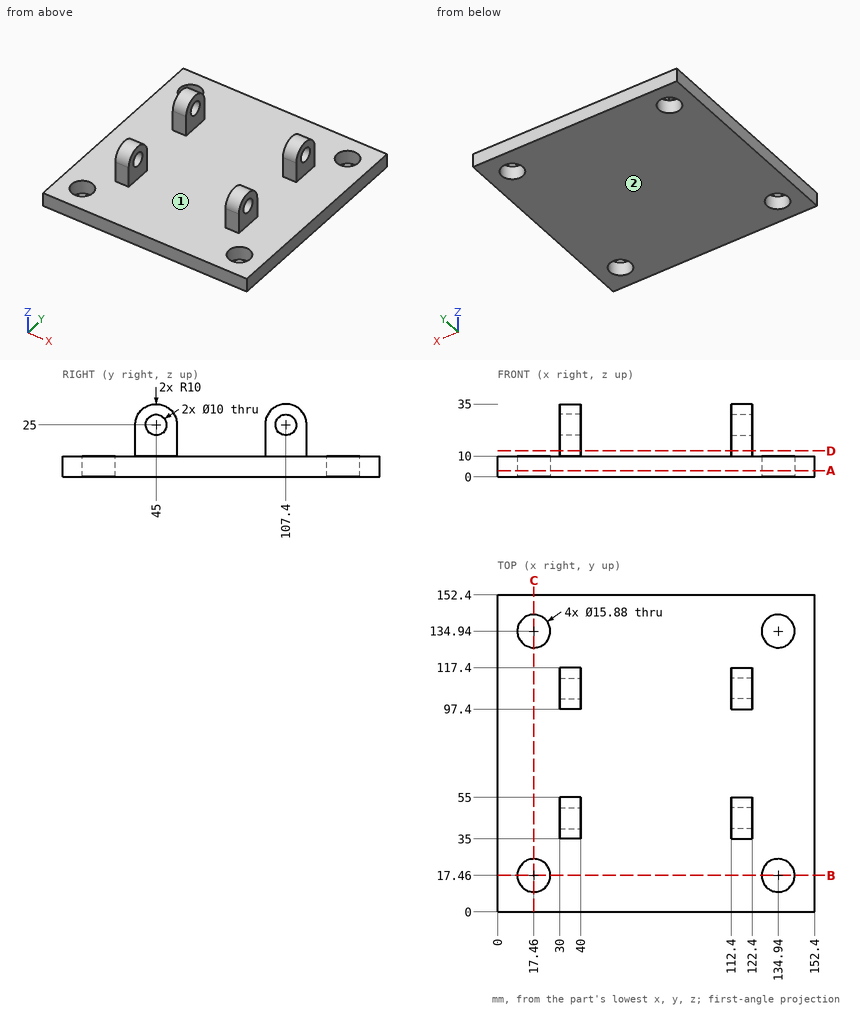
Design review of the part shown in the three views and the two pictorial views. Dimensions are in mm from the part's minimum x, y and z. Coordinates: 2 decimals unless noted, no trailing zeros. Loops run counter-clockwise (first coordinate to the right, second up) from the corner with the lowest first, then second, coordinate; pieces in that order, holes last.
(1) Draft analysis for pull direction X (two halves, no side actions). For the marked faces 1 and 2, state which applies: +X half, -X half, draft (parallel to the pull), parting line (faces both ways), or undercut.
Determined:
face 1: undercut
face 2: draft
(2) Insertion check: P1, Ø9.5, axis at x = 17.46, y = 17.46, coming from the -Z side; P2, Ø6, axis at y = 41, z = 26, coming from the -X side; P3, Ø16, axis at y = 45, z = 25, coming from the +X side; P4, Ø11, axis at x = 117.5, z = 17, coming from the +Y side. Each pin has a flat end and moves straight along its axis. Give the tip position at first contact, or say it passes through.
Determined:
P1: passes through
P2: stops at x = 30
P3: stops at x = 122.4
P4: stops at y = 117.4
(3) Consider section A-A, the plane z = 3. Give the boundary of the cut face in (x, y), plus the area to 3 significant figures.
Determined:
outline: (0, 0) - (152.4, 0) - (152.4, 152.4) - (0, 152.4) - close; hole circle Ø15.88 at (17.46, 17.46); hole circle Ø15.88 at (17.46, 134.94); hole circle Ø15.88 at (134.94, 17.46); hole circle Ø15.88 at (134.94, 134.94)
area: 22,400 mm2
(4) Consider section B-B, the plane y = 17.46. Give the boundary of the cut face in (x, z).
Determined:
outline: (0, 0) - (9.52, 0) - (9.52, 10) - (0, 10) - close; (25.4, 0) - (127, 0) - (127, 10) - (25.4, 10) - close; (142.88, 0) - (152.4, 0) - (152.4, 10) - (142.88, 10) - close
(5) Consider section D-D, the plane z = 12.5. Give the boundary of the cut face in (x, y), plus the area to 3 significant figures.
Determined:
outline: (30, 35) - (40, 35) - (40, 55) - (30, 55) - close; (30, 97.4) - (40, 97.4) - (40, 117.4) - (30, 117.4) - close; (112.4, 35) - (122.4, 35) - (122.4, 55) - (112.4, 55) - close; (112.4, 97.4) - (122.4, 97.4) - (122.4, 117.4) - (112.4, 117.4) - close
area: 800 mm2
(6) Wall thickness on L1, parallel to Y at x = 17, z = 4; L2, parallel to Y at x = 119.5, z = 25: over which ranges is each line inside the solid? List them lowest first.
Determined:
L1: y = 0 to 9.53, 25.39 to 127.01, 142.87 to 152.4
L2: y = 35 to 40, 50 to 55, 97.4 to 102.4, 112.4 to 117.4
